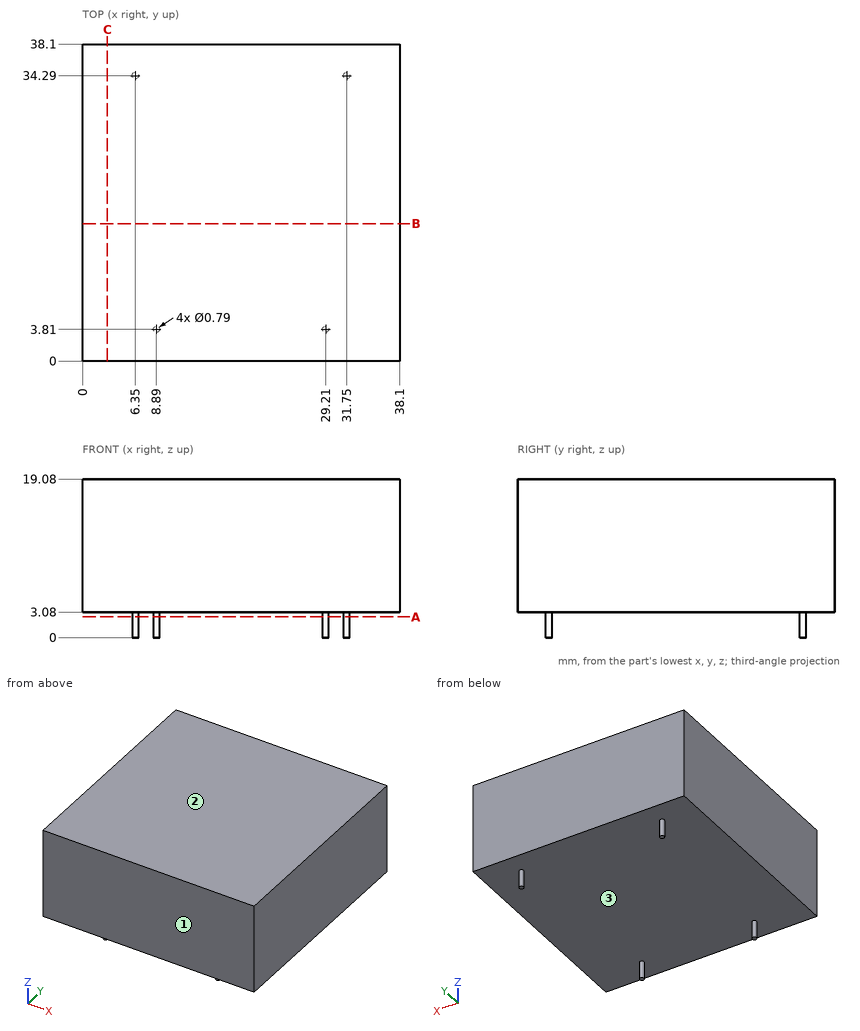
Could you check a few things on this drawing? It's one solid part, dimensions in mm from its lowest x, y, z. Coordinates: 2 decimals unless noted, no trailing zeros. Order: outer loops, then holes, each group sorted by start corner. A loop starts at its lowest first (then second) coordinate and runs counter-clockwise, first axis right, second up.
1. If we section it at A-A (z = 2.5): Please give me the cut outline in (x, y) (3 decimals), then the cut area to 3 significant figures.
2. I'm going to push flat-ended pins straight in: pin 1 (2 mm diameter, centred on x = 12.5, y = 4.5, fed in from -Z); pin 2 (10 mm diameter, centred on x = 17, z = 9.5, fed in from -Y). Where does each tip first touch, or does it pass through?
3. I need wall thicknesses on line 1 (Z direction, x = 22, y = 30). Which ranges of the line are inside material? Lowest first, please.
4. If we section it at B-B (y = 16.5): Please give me the cut outline in (x, z).
5. Thinking about a two-plate mould opening in Z: for the marked faces 1, 2 and 3, which applies, +Z half, -Z half, draft (parallel to the pull), parting line (faces both ways), or undercut?
Entries:
1. outline: circle Ø0.79 at (6.35, 34.29); circle Ø0.79 at (8.89, 3.81); circle Ø0.79 at (29.21, 3.81); circle Ø0.79 at (31.75, 34.29)
1. area: 1.96 mm2
2. pin 1: stops at z = 3.08
2. pin 2: stops at y = 0
3. line 1: z = 3.08 to 19.08
4. outline: (0, 3.08) - (38.1, 3.08) - (38.1, 19.08) - (0, 19.08) - close
5. face 1: draft
5. face 2: +Z half
5. face 3: -Z half
